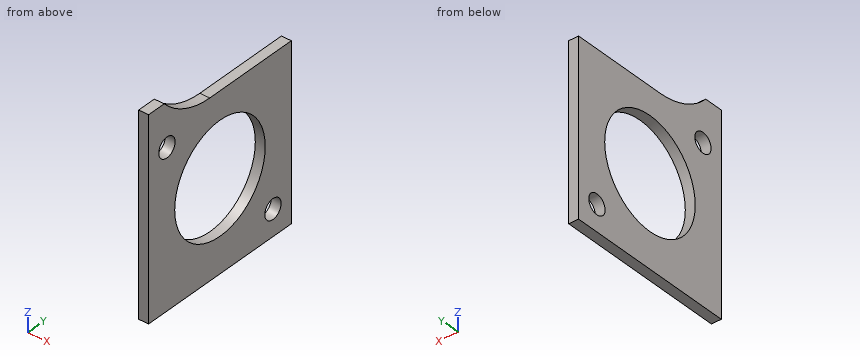
```python
from build123d import *

# Parameters (mm, degrees)
SKETCH1_R           = 2
SKETCH1_R_2         = 11.1
BOSS_EXTRUDE1_DEPTH = 2


with BuildPart() as part:
    # Sketch1 → Boss-Extrude1 (new body)
    with BuildSketch(Plane(origin=(0, 0, 0), x_dir=(0, 0, -1), z_dir=(1, 0, 0))):
        with BuildLine():
            Line((14.978419371, -24.343119081), (14.978419371, 10.656880919))
            Line((14.978419371, 10.656880919), (-20.021580629, 10.656880919))
            Line((-20.021580629, 10.656880919), (-20.021580629, -9.343119081))
            ThreePointArc((-20.021580629, -9.343119081), (-21.328516692, -15.466843438), (-25.021580629, -20.523458968))
            Line((-25.021580629, -20.523458968), (-25.021580629, -24.343119081))
            Line((-25.021580629, -24.343119081), (14.978419371, -24.343119081))
        make_face()
        with Locations((9.692898744, 6.156880919)):
            Circle(SKETCH1_R, mode=Mode.SUBTRACT)
        with Locations((-16.307101256, -19.843119081)):
            Circle(SKETCH1_R, mode=Mode.SUBTRACT)
        with Locations((-3.307101256, -6.843119081)):
            Circle(SKETCH1_R_2, mode=Mode.SUBTRACT)
    extrude(amount=BOSS_EXTRUDE1_DEPTH)


solid = part.part
```
Read the model definition and answer for the solid it produces. Units are mm, in the model's axes. Give positions to 0.01 mm unless a question says otherwise; leave off trailing zeros. Order: outer loops, then holes, each group sorted by start corner. A loop starts at its lowest first (then second) coordinate and runs counter-clockwise, first axis right, second up.
(1) Find section B-B (y = -14). Give the vertices of the cut face in (x, z).
(2) Find section A-A (z = -10). Give the vertices of the cut face in (x, y), plus the area to 3 significant figures.
(3) Straight lines are drawn through the part: L1, parallel to Z at x = 1.75, y = -7; L2, parallel to Z at x = 0.1, y = -13; L3, parallel to Y at x = 1.75, z = -3. For each, find the intervals that lie inside material, in ascending order.
(4) Given pin 1 (5 mm diameter, centred on y = -12, z = 20, fed in from -X); pin 2 (1 mm diameter, centred on x = 0.5, y = 1, fed in from +Z); pin 3 (20 mm diameter, centred on y = -6.84, z = 3.31, fed in from +X) (1 decimal); pin 4 (1 mm diameter, centred on x = 1.5, y = -16.5, fed in from +Z), each flat-ended and moving along its own axis, determine where each tip first touches the part or whether it passes through.
(5) Find section C-C (x = 0.7). Give the vertices of the cut face in (y, z).
Result sheet:
1. outline: (0, -14.98) - (2, -14.98) - (2, -5.18) - (0, -5.18) - close; (0, 11.79) - (2, 11.79) - (2, 20.76) - (0, 20.76) - close
2. outline: (0, -24.34) - (2, -24.34) - (2, 4.18) - (0, 4.18) - close; (0, 8.13) - (2, 8.13) - (2, 10.66) - (0, 10.66) - close
2. area: 62.1 mm2
3. L1: z = -14.98 to -7.79, 14.41 to 20.02
3. L2: z = -14.98 to -5.93, 12.54 to 20.47
3. L3: y = -24.34 to -15.98, 2.29 to 10.66
4. pin 1: stops at x = 0
4. pin 2: stops at z = 20.02
4. pin 3: passes through
4. pin 4: stops at z = 22.12
5. outline: (-24.34, -14.98) - (10.66, -14.98) - (10.66, 20.02) - (-9.34, 20.02) arc R15 cw to (-20.52, 25.02) - (-24.34, 25.02) - close; hole circle Ø4 at (-19.84, 16.31); hole circle Ø22.2 at (-6.84, 3.31); hole circle Ø4 at (6.16, -9.69)
